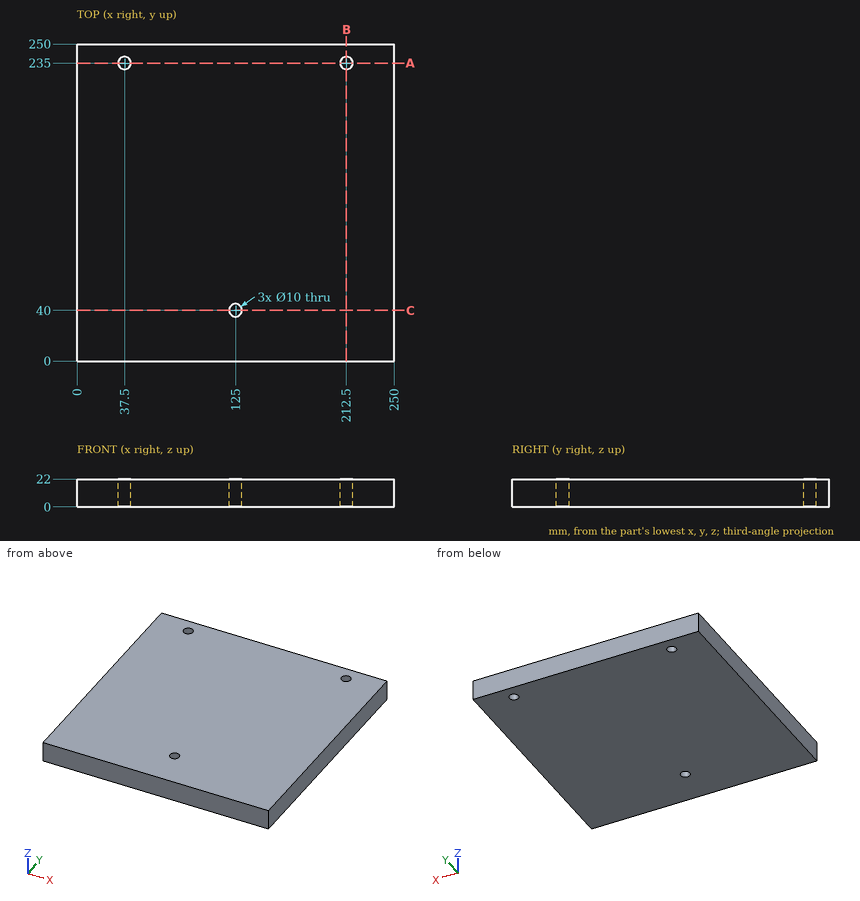
Job drawing, mm, ordinate dimensions from the low corner. One solid piece. Give positions to 0.01 mm unless a question says otherwise; leave off trailing zeros. Write each loop counter-clockwise with the first axis right and the second up, starting at its lowest first coordinate (ties: lowest second). Pieces come first, ordered by that corner, then holes. Notation, with made-up numbers: M 85,-21 L 120,-21 A15 ccw 120,0 Z; hole C -25,89 d11. An arc over 180 degrees is marked long. One line per item, written item: value. Start each with the question number.
Q1. Saw through at B-B, the plane x = 212.5. Write the cut outline in (y, z), plus the area to 3 significant figures.
Q2. Drop flat-ended pins along their axis: pin 1 Ø10 at (y, z) = (103, 10) entering from -X; pin 2 Ø9 at (x, y) = (125, 40) entering from -Z. Give the stop position or say it passes through.
Q3. Saw through at C-C, the plane y = 40. Write the cut outline in (x, z).
Q4. Probe probe 1 along Y at (x, z) = (37.5, 7.5); probe 2 along X at (y, z) = (234, 17.25); probe 3 along X at (y, z) = (43, 13). List the from-to ranges inside material, lowest first. Write a range as [from, to].
Q5. Saw through at A-A, the plane y = 235. Write the cut outline in (x, z).
Output values:
1. outline: M 0,0 L 230,0 L 230,22 L 0,22 Z; M 240,0 L 250,0 L 250,22 L 240,22 Z
1. area: 5,280 mm²
2. pin 1: stops at x = 0
2. pin 2: passes through
3. outline: M 0,0 L 120,0 L 120,22 L 0,22 Z; M 130,0 L 250,0 L 250,22 L 130,22 Z
4. probe 1: y = [0, 230], [240, 250]
4. probe 2: x = [0, 32.6], [42.4, 207.6], [217.4, 250]
4. probe 3: x = [0, 121], [129, 250]
5. outline: M 0,0 L 32.5,0 L 32.5,22 L 0,22 Z; M 42.5,0 L 207.5,0 L 207.5,22 L 42.5,22 Z; M 217.5,0 L 250,0 L 250,22 L 217.5,22 Z
